```python
from build123d import *

# Parameters (mm, degrees)
F0_W = 2.1742532432
F0_H = 0.9419020339


# Not quite as in the source:
# - ends of sketch curves that miss each other by under 0.0002 mm in the source are joined
# - the dataset's text gives a spline's control points without its knots; the knots are read off the source's solid


with BuildPart() as f1:
    # F0 (on Front) → F1 (revolve)
    with BuildSketch(Plane.XZ):
        with BuildLine():
            Line((30.5, 90), (30.5, 4.1842871582))
            ThreePointArc((30.5, 4.1842871582), (29.2386865937, 1.7395031332), (26.5153540474, 1.3504783524))
            add(Edge.make_bspline(
                [(28.6535172577, 0.6161086402), (27.9351354208, 0.8594614999), (27.2238062641, 1.1043168589), (26.5153540474, 1.3504783524)],
                knots=[0.0654689301, 0.0654689301, 0.0654689301, 0.0654689301, 0.1426249603, 0.1426249603, 0.1426249603, 0.1426249603], degree=3))
            ThreePointArc((28.6535172577, 0.6161086402), (30.5321765876, 1.9778408883), (31.25, 4.1842871582))
            Line((31.25, 4.1842871582), (31.25, 90.000003855))
            add(Edge.make_bspline(
                [(31.25, 90.000003855), (31.2499948057, 91.0105522306), (31.0401649353, 93.1352024306), (29.9495012867, 97.7430729313), (27.5987257036, 104.0623990971), (24.0115192635, 112.0918752945), (20.4584738513, 120.0703885968), (17.7582794948, 127.4728481178), (15.2441676605, 137.0543853988), (14.4983428208, 144.4691488625), (14.4499999999, 150.0032696799)],
                knots=[0, 0, 0, 0, 0.0625, 0.125, 0.25, 0.375, 0.5, 0.625, 0.75, 0.9999509591, 0.9999509591, 0.9999509591, 0.9999509591], degree=3))
            Line((14.45, 150.0032696799), (14.45, 150.9451717138))
            Line((14.45, 150.9451717138), (14.45, 171.3955121697))
            Line((14.45, 171.3955121697), (13.7, 171.3955121697))
            Line((13.7, 171.3955121697), (13.7, 150))
            add(Edge.make_bspline(
                [(30.5, 90), (30.4999601958, 97.7439469245), (17.5798622294, 121.2385566117), (13.7960969357, 138.9584630881), (13.7, 150)],
                knots=[0, 0, 0, 0, 0.5049991048, 1, 1, 1, 1], degree=3))
        make_face()
        with BuildLine():
            add(Edge.make_bspline(
                [(28.6535172577, 0.6161086402), (27.9351354208, 0.8594614999), (27.2238062641, 1.1043168589), (26.5153540474, 1.3504783524)],
                knots=[0.0654689301, 0.0654689301, 0.0654689301, 0.0654689301, 0.1426249603, 0.1426249603, 0.1426249603, 0.1426249603], degree=3))
            add(Edge.make_bspline(
                [(26.5153540474, 1.3504783524), (23.505060911, 2.3964462197), (15.7684223832, 5.1935195764), (6.1960769817, 8.0488463864), (0, 8)],
                knots=[0.1426249603, 0.1426249603, 0.1426249603, 0.1426249603, 0.4704696092, 1, 1, 1, 1], degree=3))
            Line((0, 8), (0.0059123945, 7.2500233046))
            add(Edge.make_bspline(
                [(26.2691917605, 0.6420238521), (25.2813726049, 0.9852492871), (23.1576852685, 1.73281816), (20.4345242005, 2.6915237158), (18.0535614936, 3.508219), (15.6035591078, 4.32926986), (12.4109579359, 5.3369129826), (7.0731993079, 6.7140944287), (2.8622270402, 7.272540883), (0.0059123945, 7.2500233046)],
                knots=[0.1426251828, 0.1426251828, 0.1426251828, 0.1426251828, 0.25, 0.375, 0.4375, 0.5, 0.625, 0.75, 1, 1, 1, 1], degree=3))
            ThreePointArc((26.2691917605, 0.6420238521), (27.4592400633, 0.4345086811), (28.6535172577, 0.6161086402))
        make_face()
        with Locations((15.5371266216, 150.4742206969)):
            Rectangle(F0_W, F0_H)
    revolve(axis=Axis((0.0029561972, 0, 7.6250116523), (0.0078831927, 0, -0.9999689272)))


solid = f1.part
```
Verification items for the finished model (mm, model axes). A direction names the side the tool comes from. Give positions to 0.01 mm unless a question says otherwise; leave off trailing zeros. Use a Markdown table: item, result.
1) Mould release check, pull along X, two halves, no side actions. Record for faces 3 (the conical face through (-14.201, -11.994, 150.133)), 4 (the conical face through (6.809, -12.566, 160.494)): pulls with the +X half, pulls with the -X half, needs draft (parallel to the pull), parting line crosses it, or undercut.
Results:
| item | result |
|---|---|
| face 3 | parting line crosses it |
| face 4 | undercut |
2) Tool access check on faces 1 (the conical face through (28.15, 11.8, 46.47)), 2 (the conical face through (14.25, 28, 47.56)). Record the directions out of +Z, -Z, +X, -X, +Y, -Y that give a thin tool (end or side, any length) a straight path to the whole face; none if there is none.
Results:
| item | result |
|---|---|
| face 1 | none |
| face 2 | -Z |
3) Depth check by flat-ended pin: pin 1 Ø2 at (y, z) = (-16, 40.5) entering from +X; pin 2 Ø8 at (y, z) = (-7.5, 145.5) entering from -X; pin 3 Ø10 at (y, z) = (22, 25) entering from +X. Enter the tip coordinate at first touch or a pass-through.
Results:
| item | result |
|---|---|
| pin 1 | x = 27.45 |
| pin 2 | x = -16.37 |
| pin 3 | x = 26.25 |
4) Material ranges on probe 1 along Y at (x, z) = (-8.5, 32.5); probe 2 along X at (y, z) = (0, 50); probe 3 along Y at (x, z) = (-19.5, 48.5), recorded low to high.
Results:
| item | result |
|---|---|
| probe 1 | -30.33 to -29.55, 29.55 to 30.33 |
| probe 2 | -31.92 to -31.17, 30.5 to 31.25 |
| probe 3 | -25.08 to -24.13, 24.13 to 25.08 |
